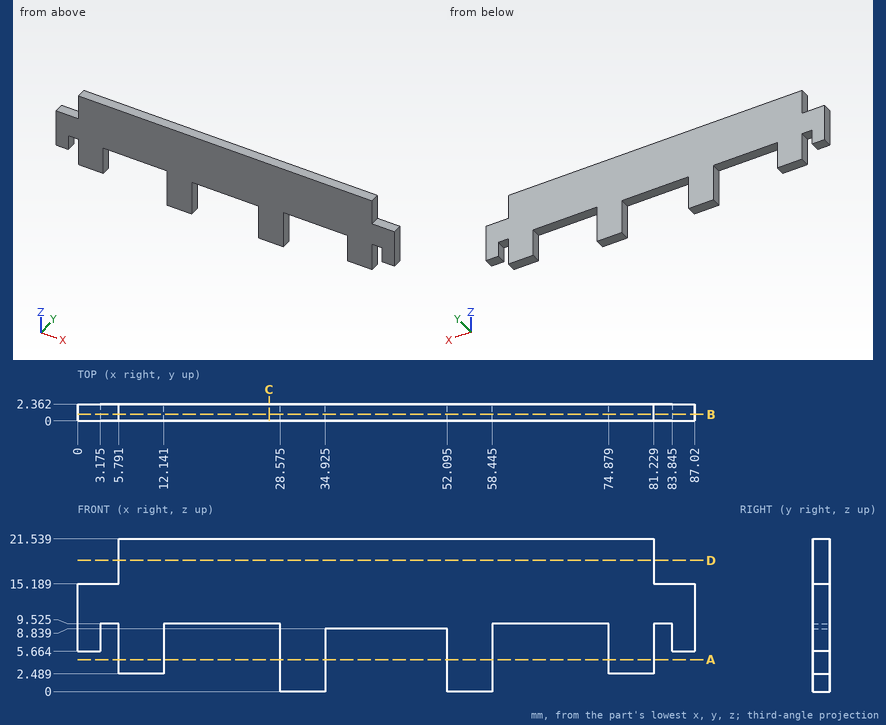
Check sheet for the drawn part. Datum: minimum x, y, z corner. Units: mm. Give positions to 0.01 mm unless a question says otherwise; leave off trailing zeros. Order: outer loops, then holes, each group sorted by start corner. A loop starts at its lowest first (then second) coordinate and runs counter-clockwise, first axis right, second up. Notation, with made-up numbers: (-1.75, 35.5) -> (30.25, 35.5) arc R19 ccw to (30.25, 40.5) -> close; hole circle Ø6 at (85, 42.5). An arc over 180 degrees is marked (long way). Return JSON: item names as keys, results as strings.
1. Cross-section at C-C, the plane x = 27. Record the cut outline in (y, z) (1 decimal), plus the area to 3 significant figures.
From the geometry:
{"outline": "(0, 9.5) -> (2.4, 9.5) -> (2.4, 21.5) -> (0, 21.5) -> close", "area": "28.4 mm^2"}
2. Cross-section at A-A, the plane z = 4.5. Record the cut outline in (x, y) (1 decimal).
From the geometry:
{"outline": "(5.8, 0) -> (12.1, 0) -> (12.1, 2.4) -> (5.8, 2.4) -> close; (28.6, 0) -> (34.9, 0) -> (34.9, 2.4) -> (28.6, 2.4) -> close; (52.1, 0) -> (58.4, 0) -> (58.4, 2.4) -> (52.1, 2.4) -> close; (74.9, 0) -> (81.2, 0) -> (81.2, 2.4) -> (74.9, 2.4) -> close"}
3. Cross-section at B-B, the plane y = 0.9. Record the cut outline in (x, z) (1 decimal), plus the area to 3 significant figures.
From the geometry:
{"outline": "(0, 5.7) -> (3.2, 5.7) -> (3.2, 9.5) -> (5.8, 9.5) -> (5.8, 2.5) -> (12.1, 2.5) -> (12.1, 9.5) -> (28.6, 9.5) -> (28.6, 0) -> (34.9, 0) -> (34.9, 8.8) -> (52.1, 8.8) -> (52.1, 0) -> (58.4, 0) -> (58.4, 9.5) -> (74.9, 9.5) -> (74.9, 2.5) -> (81.2, 2.5) -> (81.2, 9.5) -> (83.8, 9.5) -> (83.8, 5.7) -> (87, 5.7) -> (87, 15.2) -> (81.2, 15.2) -> (81.2, 21.5) -> (5.8, 21.5) -> (5.8, 15.2) -> (0, 15.2) -> close", "area": "1,220 mm^2"}
4. Go/stop test with flat-tipped pins: P1, Ø0.7, axis at y = 1, z = 4.5, coming from the -X side; P2, Ø1.2, axis at x = 46, y = 1, coming from the -Z side; P3, Ø1.2, axis at y = 1, z = 18, coming from the +X side. Record where each tip stops, or that it passes through.
From the geometry:
{"P1": "x = 5.79", "P2": "z = 8.84", "P3": "x = 81.23"}
5. Material ranges on probe 1 along X at (y, z) = (2.25, 7.5) (1 decimal); probe 2 along X at (y, z) = (2.1, 4.25) (1 decimal); probe 3 along X at (y, z) = (1.45, 1.75) (1 decimal), recorded low to high. Write a range as [from, to].
From the geometry:
{"probe 1": "[0, 3.2], [5.8, 12.1], [28.6, 34.9], [52.1, 58.4], [74.9, 81.2], [83.8, 87]", "probe 2": "[5.8, 12.1], [28.6, 34.9], [52.1, 58.4], [74.9, 81.2]", "probe 3": "[28.6, 34.9], [52.1, 58.4]"}
6. Cross-section at D-D, the plane z = 18.5. Record the cut outline in (x, y), plus the area to 3 significant figures.
From the geometry:
{"outline": "(5.79, 0) -> (81.23, 0) -> (81.23, 2.36) -> (5.79, 2.36) -> close", "area": "178 mm^2"}
